from build123d import *

# Parameters (mm, degrees)
SKETCH_2_R               = 1.6
CUT_EXTRUDE_1_DEPTH      = 8
PATTERN_CIRCULAR_1_COUNT = 8
SKETCH_3_R               = 1.6
CUT_EXTRUDE_2_DEPTH      = 10
SKETCH_4_R               = 3
CUT_EXTRUDE_6_DEPTH      = 3
PATTERN_CIRCULAR_2_COUNT = 8
SKETCH_5_R               = 3
CUT_EXTRUDE_7_DEPTH      = 1
PATTERN_CIRCULAR_3_COUNT = 3
CHAMFER_1_SIZE           = 2


with BuildPart() as part:
    # 草图1 → 旋转1 (revolve)
    with BuildSketch(Plane.XY, mode=Mode.PRIVATE) as revolve_1_sk:
        Polygon((-14, 0), (-16.6, 0), (-16.6, 3), (-22.6, 3), (-22.6, 9), (-16.6, 9), (-16.6, 28), (-6.75, 28), (-6.75, 25), (-14, 25), align=None)
    revolve(revolve_1_sk.sketch.rotate(Axis((0, 0, 0), (0, 1, 0)), 270), axis=Axis((0, 0, 0), (0, 1, 0)))

    # 草图2 → 切除-拉伸1 (cut)
    with BuildSketch(Plane.XZ.offset(-3)):
        with Locations(Location((0, -20, 0), (0, 0, 270))):
            Circle(SKETCH_2_R)
    cut_extrude_1 = extrude(amount=-CUT_EXTRUDE_1_DEPTH, mode=Mode.SUBTRACT)

    # 阵列(圆周)1: 切除-拉伸1 ×8 about axis
    pattern_circular_1_axis = Axis((0, 0, 0), (0, 1, 0))
    for i in range(1, PATTERN_CIRCULAR_1_COUNT):
        add(cut_extrude_1.rotate(pattern_circular_1_axis, i * 360 / PATTERN_CIRCULAR_1_COUNT), mode=Mode.SUBTRACT)

    # 草图3 → 切除-拉伸2 (cut)
    with BuildSketch(Plane(origin=(0, 28, 0), x_dir=(1, 0, 0), z_dir=(0, 1, 0))):
        with Locations(Location((0, -9.5, 0), (0, 0, 270))):
            Circle(SKETCH_3_R)
        with Locations(Location((-8.227241336, 4.75, 0), (0, 0, 270))):
            Circle(SKETCH_3_R)
        with Locations(Location((8.227241336, 4.75, 0), (0, 0, 270))):
            Circle(SKETCH_3_R)
    extrude(amount=-CUT_EXTRUDE_2_DEPTH, mode=Mode.SUBTRACT)

    # 草图4 → 切除-拉伸6 (cut)
    with BuildSketch(Plane(origin=(0, 9, 0), x_dir=(1, 0, 0), z_dir=(0, 1, 0))):
        with Locations((20, 0)):
            Circle(SKETCH_4_R)
    cut_extrude_6 = extrude(amount=-CUT_EXTRUDE_6_DEPTH, mode=Mode.SUBTRACT)

    # 阵列(圆周)2: 切除-拉伸6 ×8 about axis
    pattern_circular_2_axis = Axis((0, 0, 0), (0, 1, 0))
    for i in range(1, PATTERN_CIRCULAR_2_COUNT):
        add(cut_extrude_6.rotate(pattern_circular_2_axis, i * 360 / PATTERN_CIRCULAR_2_COUNT), mode=Mode.SUBTRACT)

    # 草图5 → 切除-拉伸7 (cut)
    with BuildSketch(Plane(origin=(0, 28, 0), x_dir=(1, 0, 0), z_dir=(0, 1, 0))):
        with Locations((8.227241336, 4.75)):
            Circle(SKETCH_5_R)
    cut_extrude_7 = extrude(amount=-CUT_EXTRUDE_7_DEPTH, mode=Mode.SUBTRACT)

    # 阵列(圆周)3: 切除-拉伸7 ×3 about axis
    pattern_circular_3_axis = Axis((0, 0, 0), (0, 1, 0))
    for i in range(1, PATTERN_CIRCULAR_3_COUNT):
        add(cut_extrude_7.rotate(pattern_circular_3_axis, i * 360 / PATTERN_CIRCULAR_3_COUNT), mode=Mode.SUBTRACT)

    # 倒角1
    # the kernel refuses this chamfer: 2 mm, written as the material it adds along each edge
    with BuildSketch(Plane(origin=(0, 9, 0), x_dir=(0, 0, -1), z_dir=(1, 0, 0))) as chamfer_1_piece_1_section:
        Polygon((16.6 + CHAMFER_1_SIZE, 0), (16.6, CHAMFER_1_SIZE), (16.6, 0), align=None)
    chamfer_1_piece_1 = revolve(axis=Axis((0, 9, 0), (0, 1, 0)), mode=Mode.PRIVATE)
    chamfer_1_piece_1 = chamfer_1_piece_1 - Plane(origin=(-14.142135624, 9.253857846, 14.142135624), x_dir=(-0.7071067811865477, 0, 0.7071067811865475), z_dir=(0, 1, 0)) * Cylinder(3, 75, mode=Mode.PRIVATE)
    chamfer_1_piece_1 = chamfer_1_piece_1 - Plane(origin=(20, 9.253857846, 0), x_dir=(1, 0, 0), z_dir=(0, 1, 0)) * Cylinder(3, 75, mode=Mode.PRIVATE)
    chamfer_1_piece_1 = chamfer_1_piece_1 - Plane(origin=(14.142135624, 9.253857846, 14.142135624), x_dir=(0.7071067811865474, 0, 0.7071067811865477), z_dir=(0, 1, 0)) * Cylinder(3, 75, mode=Mode.PRIVATE)
    chamfer_1_piece_1 = chamfer_1_piece_1 - Plane(origin=(0, 9.253857846, 20), x_dir=(0, 0, 1), z_dir=(0, 1, 0)) * Cylinder(3, 75, mode=Mode.PRIVATE)
    chamfer_1_piece_1 = chamfer_1_piece_1 - Plane(origin=(-20, 9.253857846, 0), x_dir=(-1, 0, 0), z_dir=(0, 1, 0)) * Cylinder(3, 75, mode=Mode.PRIVATE)
    chamfer_1_piece_1 = chamfer_1_piece_1 - Plane(origin=(-14.142135624, 9.253857846, -14.142135624), x_dir=(-0.7071067811865475, 0, -0.7071067811865476), z_dir=(0, 1, 0)) * Cylinder(3, 75, mode=Mode.PRIVATE)
    chamfer_1_piece_1 = chamfer_1_piece_1 - Plane(origin=(0, 9.253857846, -20), x_dir=(0, 0, -1), z_dir=(0, 1, 0)) * Cylinder(3, 75, mode=Mode.PRIVATE)
    chamfer_1_piece_1 = chamfer_1_piece_1 - Plane(origin=(14.142135624, 9.253857846, -14.142135624), x_dir=(0.7071067811865476, 0, -0.7071067811865475), z_dir=(0, 1, 0)) * Cylinder(3, 75, mode=Mode.PRIVATE)
    add(chamfer_1_piece_1)
    # the kernel refuses this chamfer: 2 mm, written as the material it takes off along each edge
    with BuildSketch(Plane(origin=(0, 28, 0), x_dir=(0, 0, -1), z_dir=(1, 0, 0))) as chamfer_1_2_piece_1:
        Polygon((16.6 - CHAMFER_1_SIZE, 0), (16.6, -CHAMFER_1_SIZE), (16.6, 0), align=None)
    revolve(axis=Axis((0, 28, 0), (0, 1, 0)), mode=Mode.SUBTRACT)


solid = part.part
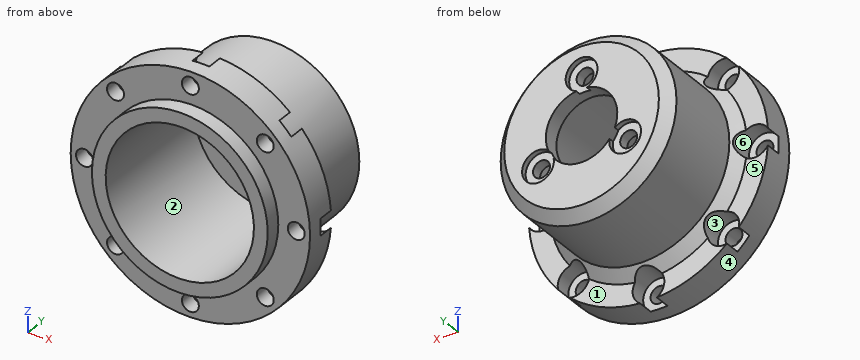
Input: part model. Units: mm. Frame: model coordinates. Face numbers are marked on the shaded views. A direction names the side the tool comes from. Coordinates: 2 decimals unless noted, no trailing zeros. Loops run counter-clockwise (first coordinate to the right, second up) from the corner with the lowest first, then second, coordinate; pieces in that order, holes last. Notation, with made-up numbers: (42, 4) - (53, 4) arc R14 cw to (53, 28) - close; hole circle Ø4 at (74.25, -15.5). An arc over 180 degrees is marked (long way). Answer in a Markdown table with one row per item. Add a question column.
Item 1: Section query D-D on x = -20. Return the cut outline in (y, z), then the cut area to 3 significant figures.
Item 2: Line query: line 1 along Z through (x, y) = (-14.5, 5.75); line 2 along Z through (x, y) = (12, 6.5); line 3 along Y through (x, z) = (1, 11.5). Output: solid intervals per line, ascending. Write a range as [from, to].
Item 3: Section query A-A on z = 0. State how many separate pieces and enclosed holes the cut face has, then the cut area to 3 significant figures.
Item 4: Section query C-C on z = 20. Return the cut outline in (x, y).
Item 5: Contact query for flat-ended pins moving along their axis: P1, Ø1.5, axis at y = 23.5, z = -14.5, coming from the +X side; P2, Ø4, axis at x = 8, z = -17.5, coming from the +Y side; P3, Ø8, axis at x = 6.5, y = 23, coming from the +Z side; P4, Ø2.5, axis at x = 14.14, z = 14.14, coming from the -Y side. Output: stop coordinate, or through.
Item 6: Mould query, pull axis Z, two halves, no side actions, for the marked faces 4, 5 and 6. Classes: released by +Z, released by -Z, zero draft, split by the parting line, or undercut.
Item 7: Access query for the marked faces 1, 2 and 3. Directions: +Z, -Z, +X, -X, +Y, -Y. A direction counts if a zero-diameter tool reaches every point of the face in a straight line with its end or side. Return the directions, or none.
Recorded:
| question | item | result |
|---|---|---|
| 1 | outline | (3, -10.52) - (9, -10.52) - (9, -3) - (6, -3) - (6, -1.6) - (3, -1.6) - close; (3, 1.6) - (6, 1.6) - (6, 3) - (9, 3) - (9, 10.52) - (3, 10.52) - close |
| 1 | area | 98.7 mm^2 |
| 2 | line 1 | [-17.34, -15.7], [-12.58, 12.58], [15.7, 17.34] |
| 2 | line 2 | [-19.15, -16.24], [-12.04, -7.21], [7.21, 12.04], [16.24, 19.15] |
| 2 | line 3 | [25, 27] |
| 3 | separate pieces | 4 |
| 3 | enclosed holes | 0 |
| 3 | area | 206 mm^2 |
| 4 | outline | (-10.52, 3) - (-1.6, 3) - (-1.6, 6) - (-3, 6) - (-3, 9) - (-10.52, 9) - close; (1.6, 3) - (10.52, 3) - (10.52, 9) - (3, 9) - (3, 6) - (1.6, 6) - close |
| 5 | P1 | x = 9.3 |
| 5 | P2 | y = 10.36 |
| 5 | P3 | z = 16.41 |
| 5 | P4 | through |
| 6 | face 4 | split by the parting line |
| 6 | face 5 | zero draft |
| 6 | face 6 | undercut |
| 7 | face 1 | -Z, +X, +Y |
| 7 | face 2 | -Y |
| 7 | face 3 | +Y |
